from build123d import *

# Parameters (mm, degrees)
ESBO_O1_R                = 6.35
ESBO_O1_R_2              = 3.25
RESSALTO_EXTRUS_O1_DEPTH = 15
ESBO_O2_W                = 20
ESBO_O2_H                = 3.1
RESSALTO_EXTRUS_O2_DEPTH = 30


with BuildPart() as part:
    # Esboço1 → Ressalto-extrusão1 (new, symmetric)
    with BuildSketch(Plane.XY):
        Circle(ESBO_O1_R)
        Circle(ESBO_O1_R_2, mode=Mode.SUBTRACT)
    extrude(amount=RESSALTO_EXTRUS_O1_DEPTH, both=True)

    # Esboço2 → Ressalto-extrusão2 (add)
    with BuildSketch(Plane.XY.offset(15)):
        with Locations((10, -4.8)):
            Rectangle(ESBO_O2_W, ESBO_O2_H)
    extrude(amount=-RESSALTO_EXTRUS_O2_DEPTH)


solid = part.part
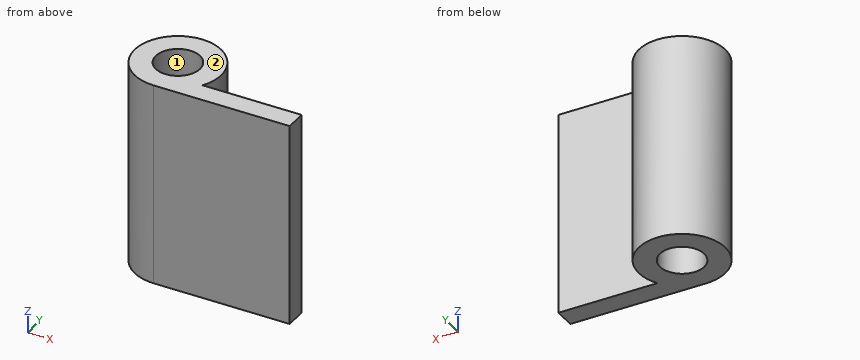
Source: CAD feature listing. Evaluate the final solid. Frame: model axes, mm. Face numbers are marked on the shaded views. Coordinates: 2 decimals unless noted, no trailing zeros. Loops run counter-clockwise (first coordinate to the right, second up) from the corner with the lowest first, then second, coordinate; pieces in that order, holes last. Notation, with made-up numbers: (30.5, 79.25) -> (86.5, 79.25) arc R15 ccw to (86.5, 98.25) -> close; hole circle Ø1 at (-12, 50). An arc over 180 degrees is marked (long way). Answer in a Markdown table with one row per item. Add a question column.
Q1. Ray query, line 1 along X through (y, z) = (0, -6); line 2 along X through (y, z) = (1.75, 9.75). Return the intervals inside material, ascending.
Q2. Pull-direction query (X, two-part tool) for the marked faces 1 and 2; classes: pulls with the +X half, pulls with the -X half, needs draft (parallel to the pull), parting line crosses it, or undercut.
Q3. Section C-C on x = 5. Return the cut outline in (y, z).
Q4. Contact query for flat-ended pins moving along their axis: pin 1 Ø1 at (y, z) = (5, 10.5) entering from -X; pin 2 Ø11.5 at (x, z) = (14, -4) entering from +Y. Output: stop coordinate, or through.
Q5. Section A-A on y = 0. Return the cut outline in (x, z), and give its area (3 significant figures).
Q6. Section D-D on y = -2. Return the cut outline in (x, z).
Q7. Section B-B on z = 12.5. Return the cut outline in (x, y), and give its area (3 significant figures).
Computed values:
| question | item | result |
|---|---|---|
| 1 | line 1 | x = -6.35 to -3.25, 3.25 to 6.35 |
| 1 | line 2 | x = -6.1 to -2.74, 2.74 to 6.1 |
| 2 | face 1 | undercut |
| 2 | face 2 | needs draft |
| 3 | outline | (-6.35, -15) -> (3.91, -15) -> (3.91, 15) -> (-6.35, 15) -> close |
| 4 | pin 1 | stops at x = -4.48 |
| 4 | pin 2 | stops at y = -3.25 |
| 5 | outline | (-6.35, -15) -> (-3.25, -15) -> (-3.25, 15) -> (-6.35, 15) -> close; (3.25, -15) -> (6.35, -15) -> (6.35, 15) -> (3.25, 15) -> close |
| 5 | area | 186 mm^2 |
| 6 | outline | (-6.03, -15) -> (-2.56, -15) -> (-2.56, 15) -> (-6.03, 15) -> close; (2.56, -15) -> (6.03, -15) -> (6.03, 15) -> (2.56, 15) -> close |
| 7 | outline | (0, -6.35) -> (20, -6.35) -> (20, -3.25) -> (5.46, -3.25) arc R6.35 ccw (long way) to start; hole circle Ø6.5 at (0, 0) |
| 7 | area | 144 mm^2 |
